Input: part model. Units: mm. Frame: model coordinates. Face numbers are marked on the shaded views. Coordinates: 2 decimals unless noted, no trailing zeros. Loops run counter-clockwise (first coordinate to the right, second up) from the corner with the lowest first, then second, coordinate; pieces in that order, holes last.
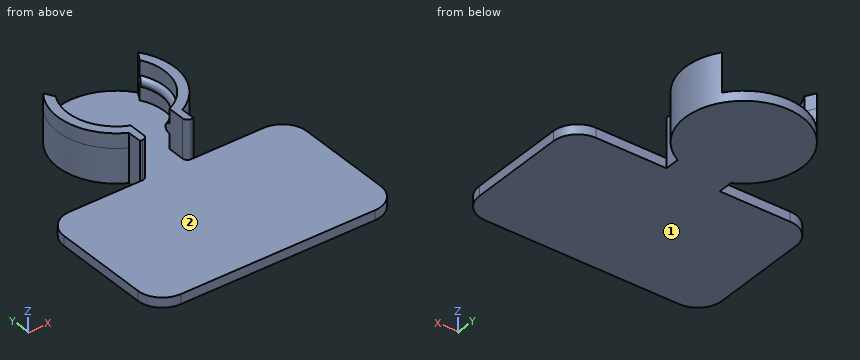
```python
from build123d import *

# Parameters (mm, degrees)
F1_DEPTH  = 2
F3_DEPTH  = 3
F5_DEPTH  = 2
F7_DEPTH  = 3
F8_R      = 0.99999
F9_W      = 20
F9_H      = 14.6653645039
F10_DEPTH = 8
F11_W     = 50
F11_H     = 30
F12_DEPTH = 2
F13_R     = 1
F14_R     = 5


# Not quite as in the source:
# - a fillet or chamfer is up to 0.001 mm smaller than in the source, because OpenCascade refuses the exact size


with BuildPart() as f1:
    # F0 (on Top) → F1 (new body)
    with BuildSketch(Plane.XY):
        with BuildLine():
            ThreePointArc((5.5, 1.5), (0, 24.1653645039), (-5.5, 1.5))
            Line((-5.5, 1.5), (-5.5, -1.5))
            ThreePointArc((-5.5, -1.5), (0, -24.1653645039), (5.5, -1.5))
            Line((5.5, -1.5), (5.5, 1.5))
        make_face()
    extrude(amount=F1_DEPTH)

    # F2 (on face) → F3 (join)
    with BuildSketch(Plane.XY.offset(2)):
        with BuildLine():
            Line((9.7844830762, 19.1125863177), (8.6602540378, 17.1653645039))
            ThreePointArc((8.6602540378, 17.1653645039), (9.4991255677, 9.0402063559), (4, 3.0002131139))
            Line((4, 3.0002131139), (4, -6.2432010007))
            Line((4, -6.2432010007), (9.1651513899, -16.1653645039))
            ThreePointArc((9.1651513899, -16.1653645039), (9.5868378212, -9.3206253964), (5.5, -3.8137179596))
            Line((5.5, -3.8137179596), (5.5, 1.5))
            ThreePointArc((5.5, 1.5), (11.6599594736, 9.3289327537), (9.7844830762, 19.1125863177))
        make_face()
        with BuildLine():
            ThreePointArc((-4, 3.0002131139), (-9.4991255677, 9.0402063559), (-8.6602540378, 17.1653645039))
            Line((-8.6602540378, 17.1653645039), (-9.7844830762, 19.1125863177))
            ThreePointArc((-9.7844830762, 19.1125863177), (-11.6599594736, 9.3289327537), (-5.5, 1.5))
            Line((-5.5, 1.5), (-5.5, -3.8137179596))
            ThreePointArc((-5.5, -3.8137179596), (-9.5868378212, -9.3206253964), (-9.1651513899, -16.1653645039))
            Line((-9.1651513899, -16.1653645039), (-4, -6.2432010007))
            Line((-4, -6.2432010007), (-4, 3.0002131139))
        make_face()
    extrude(amount=F3_DEPTH)

    # F4 (on face) → F5 (join)
    with BuildSketch(Plane.XY.offset(5)):
        with BuildLine():
            Line((-8.0717844057, 16.1461052023), (-9.7844830762, 19.1125863177))
            ThreePointArc((-9.7844830762, 19.1125863177), (-11.6599594736, 9.3289327537), (-5.5, 1.5))
            Line((-5.5, 1.5), (-5.5, -5.0414610795))
            ThreePointArc((-5.5, -5.0414610795), (-8.6043935433, -9.5263473097), (-8.5483759414, -14.980549891))
            Line((-8.5483759414, -14.980549891), (-4, -6.2432010007))
            Line((-4, -6.2432010007), (-4, 4.1031067556))
            ThreePointArc((-4, 4.1031067556), (-8.5258693153, 9.2827350759), (-8.0717844057, 16.1461052023))
        make_face()
        with BuildLine():
            ThreePointArc((5.5, 1.5), (11.6599594736, 9.3289327537), (9.7844830762, 19.1125863177))
            Line((9.7844830762, 19.1125863177), (8.0717844057, 16.1461052023))
            ThreePointArc((8.0717844057, 16.1461052023), (8.5258693153, 9.2827350759), (4, 4.1031067556))
            Line((4, 4.1031067556), (4, -6.2432010007))
            Line((4, -6.2432010007), (8.5483759414, -14.980549891))
            ThreePointArc((8.5483759414, -14.980549891), (8.6043935433, -9.5263473097), (5.5, -5.0414610795))
            Line((5.5, -5.0414610795), (5.5, 1.5))
        make_face()
    extrude(amount=F5_DEPTH)

    # F6 (on face) → F7 (join)
    with BuildSketch(Plane.XY.offset(7)):
        with BuildLine():
            Line((9.7844830762, 19.1125863177), (8.6602540378, 17.1653645039))
            ThreePointArc((8.6602540378, 17.1653645039), (9.4991255677, 9.0402063559), (4, 3.0002131139))
            Line((4, 3.0002131139), (4, -6.2432010007))
            Line((4, -6.2432010007), (9.1651513899, -16.1653645039))
            ThreePointArc((9.1651513899, -16.1653645039), (9.5868378212, -9.3206253964), (5.5, -3.8137179596))
            Line((5.5, -3.8137179596), (5.5, 1.5))
            ThreePointArc((5.5, 1.5), (11.6599594736, 9.3289327537), (9.7844830762, 19.1125863177))
        make_face()
        with BuildLine():
            ThreePointArc((-4, 3.0002131139), (-9.4991255677, 9.0402063559), (-8.6602540378, 17.1653645039))
            Line((-8.6602540378, 17.1653645039), (-9.7844830762, 19.1125863177))
            ThreePointArc((-9.7844830762, 19.1125863177), (-11.6599594736, 9.3289327537), (-5.5, 1.5))
            Line((-5.5, 1.5), (-5.5, -3.8137179596))
            ThreePointArc((-5.5, -3.8137179596), (-9.5868378212, -9.3206253964), (-9.1651513899, -16.1653645039))
            Line((-9.1651513899, -16.1653645039), (-4, -6.2432010007))
            Line((-4, -6.2432010007), (-4, 3.0002131139))
        make_face()
    extrude(amount=F7_DEPTH)

    # F8 (radius 1 in the source; OpenCascade refuses exactly that, so slightly less here)
    f8_edges = [f1.edges().sort_by_distance(p)[0] for p in [
        (8.525869, 9.282735, 7),
        (-8.525869, 9.282735, 7),
        (-8.525869, 9.282735, 5),
        (8.525869, 9.282735, 5),
        (-8.604394, -9.526347, 5),
        (-8.604394, -9.526347, 7),
        (8.604394, -9.526347, 7),
        (8.604394, -9.526347, 5),
    ]]
    fillet(f8_edges, radius=F8_R)

    # F9 (on face) → F10 (cut)
    with BuildSketch(Plane.XY.offset(10)):
        with Locations((0, -8.8326822519)):
            Rectangle(F9_W, F9_H)
    extrude(amount=-F10_DEPTH, mode=Mode.SUBTRACT)

    # F11 (on face) → F12 (join)
    with BuildSketch(Plane.XY.offset(2)):
        with Locations((0, -16.5)):
            Rectangle(F11_W, F11_H)
    extrude(amount=-F12_DEPTH)

    # F13
    f13_edges = [f1.edges().sort_by_distance(p)[0] for p in [
        (-4, -1.5, 6),
        (4, -1.5, 6),
    ]]
    fillet(f13_edges, radius=F13_R)

    # F14
    f14_edges = [f1.edges().sort_by_distance(p)[0] for p in [
        (-25, -1.5, 1),
        (-25, -31.5, 1),
        (25, -31.5, 1),
        (25, -1.5, 1),
    ]]
    fillet(f14_edges, radius=F14_R)


solid = f1.part
```
Item 1: Section query C-C (y = -2.5). Output: boundary loops of the cut face in (x, z), then the cut area to 3 significant figures.
Result:
outline: (-23, 0) - (23, 0) - (23, 2) - (-23, 2) - close
area: 92.0 mm2
Item 2: Mould query, pull axis X, two halves, no side actions, for the marked faces 1 and 2. Classes: +X half, -X half, draft (parallel to the pull), parting line (faces both ways), or undercut.
Result:
face 1: draft
face 2: undercut
Item 3: Section query B-B (z = 1). Output: boundary loops of the cut face in (x, y), then the cut area to 3 significant figures.
Result:
outline: (-25, -26.5) arc R5 ccw to (-20, -31.5) - (20, -31.5) arc R5 ccw to (25, -26.5) - (25, -6.5) arc R5 ccw to (20, -1.5) - (5.5, -1.5) - (5.5, 1.5) arc R12 ccw (long way) to (-5.5, 1.5) - (-5.5, -1.5) - (-20, -1.5) arc R5 ccw to (-25, -6.5) - close
area: 1,950 mm2
Item 4: Section query A-A (z = 8.75). Output: boundary loops of the cut face in (x, y).
Result:
outline: (-9.78, 19.11) arc R12 ccw to (-5.5, 1.5) - (-5.5, -1.5) - (-5, -1.5) arc R1 ccw to (-4, -0.5) - (-4, 3) arc R10 cw to (-8.66, 17.17) - close; (4, -0.5) arc R1 ccw to (5, -1.5) - (5.5, -1.5) - (5.5, 1.5) arc R12 ccw to (9.78, 19.11) - (8.66, 17.17) arc R10 cw to (4, 3) - close
Item 5: Contact query for flat-ended pins moving along their axis: P1, Ø2, axis at x = -11.5, z = 1.5, coming from the +Y side; P2, Ø1, axis at x = -12, y = -17.5, coming from the +Z side; P3, Ø1.4, axis at y = 1.5, z = 6, coming from the -X side. Output: stop coordinate, or through.
Result:
P1: stops at y = 17.97
P2: stops at z = 2
P3: stops at x = -6.69
Item 6: Section query D-D (x = -14). Output: boundary loops of the cut face in (y, z), then the cut area to 3 significant figures.
Result:
outline: (-31.5, 0) - (-1.5, 0) - (-1.5, 2) - (-31.5, 2) - close
area: 60.0 mm2
Item 7: Line query: L1, parallel to Z at x = -10, y = -9.5; L2, parallel to X at y = 18.5, z = 7.5; L3, parallel to X at y = 2, z = 8.75. Output: solid intervals per line, ascending.
Result:
L1: z = 0 to 2
L2: x = -10.19 to -9.43, 9.43 to 10.19
L3: x = -6.38 to -4, 4 to 6.38
